Job drawing, mm, ordinate dimensions from the low corner. One solid piece. A direction names the side the tool comes from. Give positions to 0.01 mm unless a question says otherwise; leave off trailing zeros. Write each loop counter-clockwise with the first axis right and the second up, starting at its lowest first coordinate (ties: lowest second). Pieces come first, ordered by that corner, then holes. Notation, with made-up numbers: (-5, 60) -> (32, 60) arc R27 cw to (32, 86) -> close; hole circle Ø3 at (-8, -5). An arc over 180 degrees is marked (long way). Put each result on its own line as item: value. Start each with the question number.
Item 1: Two-plate mould, pull along X, no slides. Class the marked faces 1, 2 and 3: pulls with the +X half, pulls with the -X half, needs draft (parallel to the pull), parting line crosses it, or undercut.
Item 2: Flat gauge pins, fed straight in: pin 1 Ø0.9 at (x, y) = (8.5, 0.5) entering from +Z; pin 2 Ø0.5 at (y, z) = (1.5, 8) entering from -X; pin 3 Ø2 at (x, z) = (3, 11.5) entering from +Y; pin 4 Ø0.9 at (x, y) = (9, 0.5) entering from -Z. Where does each tip first touch, or does it go through?
Item 3: Slice it at C-C, the plane x = 8.5. List the corners of the cut face in (y, z).
Item 4: Drill centre lines: line 1 along X through (y, z) = (1.35, 16); line 2 along Y through (x, z) = (4.25, 8); line 3 along X through (y, z) = (2.1, 16.25). Where is each one in solid material? Low to high.
Item 5: Slice it at D-D, the plane x = 3.5. List the corners of the cut face in (y, z).
Item 6: Slice it at A-A, the plane y = 1.3. List the corners of the cut face in (x, z).
Item 7: Slice it at B-B, the plane z = 18.75. List the corners of the cut face in (x, y), plus the area to 3 significant figures.
Item 8: Tool access for the marked faces 4 and 5: list every direction of +Z, -Z, +X, -X, +Y, -Y with a clear straight run to the whole face (end or side of a thin tool).
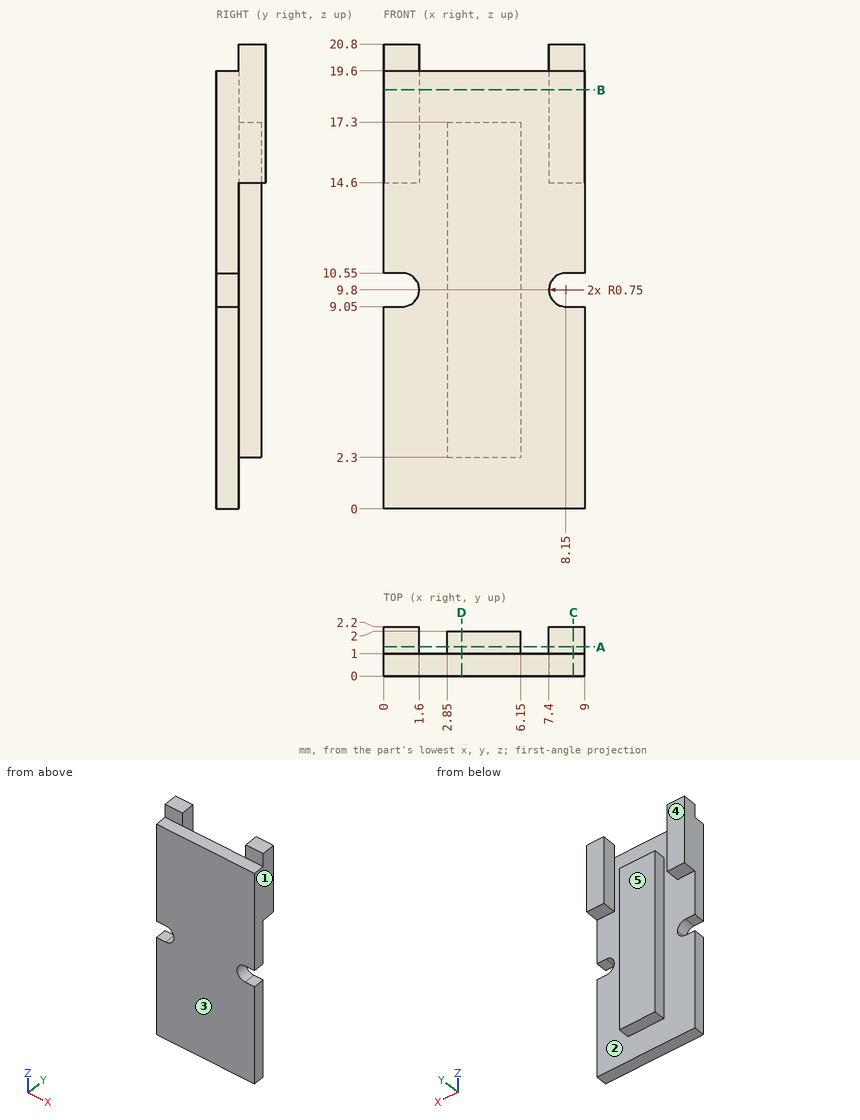
Values follow:
1. face 1: pulls with the +X half
1. face 2: undercut
1. face 3: needs draft
2. pin 1: z = 19.6
2. pin 2: x = 2.85
2. pin 3: y = 2
2. pin 4: z = 0
3. outline: (0, 0) -> (1, 0) -> (1, 9.05) -> (0, 9.05) -> close; (0, 10.55) -> (1, 10.55) -> (1, 14.6) -> (2.2, 14.6) -> (2.2, 20.8) -> (1, 20.8) -> (1, 19.6) -> (0, 19.6) -> close
4. line 1: 0 to 1.6, 2.85 to 6.15, 7.4 to 9
4. line 2: 0 to 2
4. line 3: 0 to 1.6, 7.4 to 9
5. outline: (0, 0) -> (1, 0) -> (1, 2.3) -> (2, 2.3) -> (2, 17.3) -> (1, 17.3) -> (1, 19.6) -> (0, 19.6) -> close
6. outline: (0, 14.6) -> (1.6, 14.6) -> (1.6, 20.8) -> (0, 20.8) -> close; (2.85, 2.3) -> (6.15, 2.3) -> (6.15, 17.3) -> (2.85, 17.3) -> close; (7.4, 14.6) -> (9, 14.6) -> (9, 20.8) -> (7.4, 20.8) -> close
7. outline: (0, 0) -> (9, 0) -> (9, 2.2) -> (7.4, 2.2) -> (7.4, 1) -> (1.6, 1) -> (1.6, 2.2) -> (0, 2.2) -> close
7. area: 12.8 mm2
8. face 4: +Z, -Z, +X, -X, +Y
8. face 5: +Z, -Z, +Y
